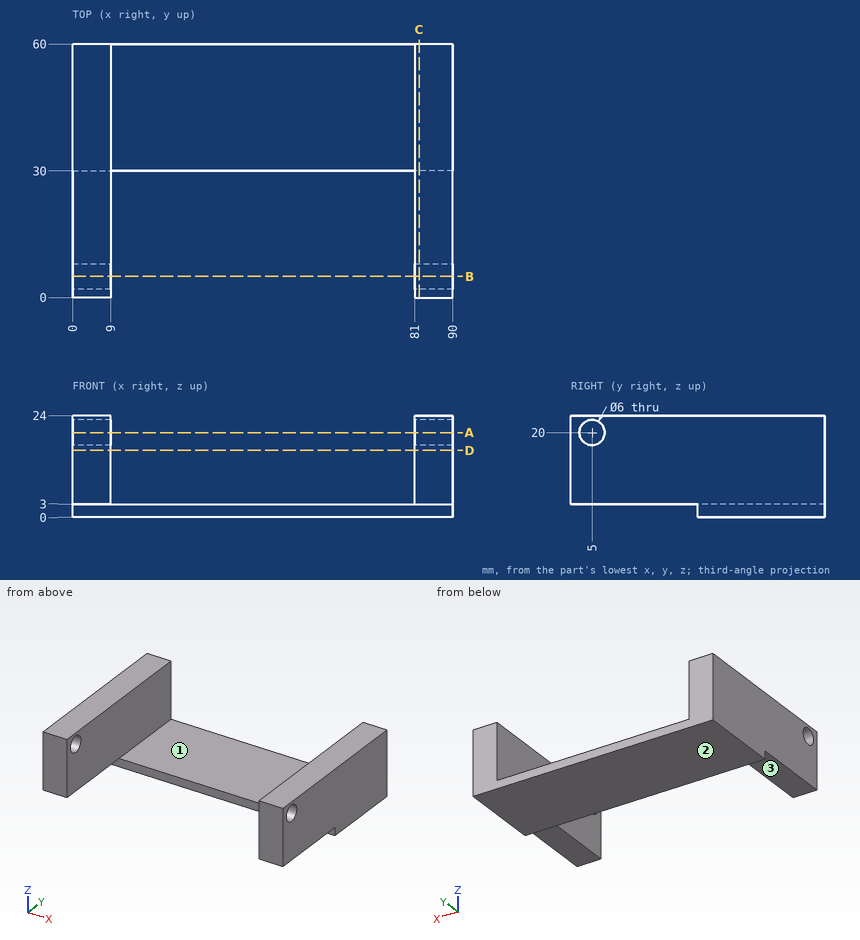
Verification items for this drawing (mm, ordinates from the low corner). A direction names the side the tool comes from. Coordinates: 2 decimals unless noted, no trailing zeros. Order: outer loops, then holes, each group sorted by start corner. A loop starts at its lowest first (then second) coordinate and runs counter-clockwise, first axis right, second up. Notation, with made-up numbers: (66, -13.75) - (104, -13.75) arc R32 cw to (104, 16.25) - close; hole circle Ø6 at (20.25, 24). An arc over 180 degrees is marked (long way). Answer in a Markdown table with one row per item. Add a question column.
1. Access from +Z, -Z, +X, -X, +Y, -Y to the whole of each face (thin tool, end or side, straight path). Record for the marked faces 1, 2 and 3.
2. Section check A-A (z = 20). Enter the section's corners in (x, y), plus the area to 3 significant figures.
3. Section check C-C (x = 82). Enter the section's corners in (y, z), plus the area to 3 significant figures.
4. Gauge pin test, flat ends, axial feed: pin 1 Ø2.5 at (x, y) = (4, 12.5) entering from -Z; pin 2 Ø2.5 at (x, z) = (43, 1.5) entering from -Y; pin 3 Ø9 at (x, y) = (38.5, 48) entering from +Z; pin 4 Ø1 at (x, z) = (75.5, 4) entering from -Y (1 decimal). Record the tip position at first contact, or that the pin passes through.
5. Section check D-D (z = 15.75). Enter the section's corners in (x, y), plus the area to 3 significant figures.
6. Material ranges on L1, parallel to Z at x = 5.5, y = 5; L2, parallel to Y at x = 85.5, z = 20; L3, parallel to X at y = 43.5, z = 22.25, recorded low to high. Write a range as [from, to].
7. Section check B-B (y = 5). Enter the section's corners in (x, z), plus the area to 3 significant figures.
Data:
| question | item | result |
|---|---|---|
| 1 | face 1 | +Z, +Y, -Y |
| 1 | face 2 | -Z, +X, -X, +Y, -Y |
| 1 | face 3 | -Z, +X, -X, -Y |
| 2 | outline | (0, 0) - (9, 0) - (9, 2) - (0, 2) - close; (0, 8) - (9, 8) - (9, 60) - (0, 60) - close; (81, 0) - (90, 0) - (90, 2) - (81, 2) - close; (81, 8) - (90, 8) - (90, 60) - (81, 60) - close |
| 2 | area | 972 mm² |
| 3 | outline | (0, 3) - (30, 3) - (30, 0) - (60, 0) - (60, 24) - (0, 24) - close; hole circle Ø6 at (5, 20) |
| 3 | area | 1,320 mm² |
| 4 | pin 1 | stops at z = 3 |
| 4 | pin 2 | stops at y = 30 |
| 4 | pin 3 | stops at z = 3 |
| 4 | pin 4 | passes through |
| 5 | outline | (0, 0) - (9, 0) - (9, 60) - (0, 60) - close; (81, 0) - (90, 0) - (90, 60) - (81, 60) - close |
| 5 | area | 1,080 mm² |
| 6 | L1 | z = [3, 17], [23, 24] |
| 6 | L2 | y = [0, 2], [8, 60] |
| 6 | L3 | x = [0, 9], [81, 90] |
| 7 | outline | (0, 3) - (9, 3) - (9, 17) - (0, 17) - close; (0, 23) - (9, 23) - (9, 24) - (0, 24) - close; (81, 3) - (90, 3) - (90, 17) - (81, 17) - close; (81, 23) - (90, 23) - (90, 24) - (81, 24) - close |
| 7 | area | 270 mm² |
